Here's how the part is built. I have some questions about the finished solid (model axes, mm). Face numbers are marked on the shaded views. A direction names the side the tool comes from. Coordinates: 2 decimals unless noted, no trailing zeros. Write each loop counter-clockwise with the first axis right and the second up, starting at its lowest first coordinate (ties: lowest second). Pieces come first, ordered by that corner, then holes.
(1) Thinking about a two-plate mould opening in X: for the marked faces 1, 2, 3 and 4, which applies, released by +X, released by -X, zero draft, split by the parting line, or undercut?
(2) Imagine slicing it at C-C, the plane y = 8. List the corners of the cut face in (x, z) for me, plus the area to 3 significant figures.
(3) For pin 1 Ø0.8 at (x, z) = (-15.5, 1.5) entering from -Y; pin 2 Ø0.8 at (y, z) = (-23, 1.5) entering from -X, each with a flat end and sliding along its axis, tell me the tip position at first contact or that it passes through.
(4) Imagine slicing it at D-D, the plane x = -14. List the corners of the cut face in (y, z) for me.
(5) Please list where these lines run through material, in increasing order: probe 1 along Y at (x, z) = (0, 1.35); probe 2 along X at (y, z) = (-25, 1.8); probe 3 along Y at (x, z) = (4, 1.9).
(6) Which directions (+Z, -Z, +X, -X, +Y, -Y) give clear straight access to the entire face, cutting with the end or side of a thin tool? Please do the marked faces 5, 6 and 7.
(7) Imagine slicing it at A-A, the plane z = 1.1. List the corners of the cut face in (x, y) for me.
(8) Imagine slicing it at B-B, the plane x = 0. List the corners of the cut face in (y, z) for me.
Autodesk Inventor part; units mm, degrees
ref_plane "YZ Plane" through (0, 0, 0) normal (1, 0, 0) x (0, 1, 0)
ref_plane "XZ Plane" through (0, 0, 0) normal (0, 1, 0) x (-1, 0, 0)
ref_plane "XY Plane" through (0, 0, 0) normal (0, 0, 1) x (1, 0, 0)
sketch "Sketch1" plane through (0, 0, 0) normal (0, 0, 1) x (1, 0, 0)
  line L0 (0, 0) -> (0, 25.4)
  line L1 (0, 0) -> (0, -25.4)
  line L2 (-19.0266, -7.6091) -> (19.0734, -7.6091)
  circle A0 centre (0, 0) radius 2.54
  circle A1 centre (0, 25.4) radius 2.54
  circle A2 centre (-19.0266, -7.6091) radius 2.54
  circle A3 centre (19.0734, -7.6091) radius 2.54
  circle A4 centre (0, -25.4) radius 2.54
  circle A5 centre (0.0234, -7.6091) radius 5.08
  arc A6 (-1.9812, -2.9413) -> (-1.7729, -1.8189) centre (-2.2521, -2.3105) ccw
  arc A7 (1.7485, -1.8423) -> (1.9483, -2.9079) centre (2.1929, -2.3105) ccw
  line L3 (-2.54, 25.4) -> (-2.54, 10.1709)
  line L4 (2.54, 25.4) -> (2.54, 10.1709)
  line L5 (-2.54, -25.4) -> (-2.54, -19.0391)
  line L6 (2.54, -25.4) -> (2.54, -19.0391)
  line L7 (19.0734, -10.1491) -> (11.43, -10.1491)
  line L8 (19.0734, -5.0691) -> (17.78, -5.0691)
  line L9 (-19.0266, -5.0691) -> (-17.78, -5.0691)
  line L10 (-19.0266, -10.1491) -> (-11.43, -10.1491)
  arc A8 (-17.78, -5.0691) -> (-2.54, 10.1709) centre (-17.78, 10.1709) ccw
  arc A9 (2.54, 10.1709) -> (17.78, -5.0691) centre (17.78, 10.1709) ccw
  arc A10 (-2.54, -19.0391) -> (-11.43, -10.1491) centre (-11.43, -19.0391) ccw
  arc A11 (11.43, -10.1491) -> (2.54, -19.0391) centre (11.43, -19.0391) ccw
  circle A12 centre (-19.0266, -7.6091) radius 1.27
  circle A13 centre (0, 25.4) radius 1.27
  circle A14 centre (19.0734, -7.6091) radius 1.27
  dimension "d0" = 25.4
  dimension "d1" = 25.4
  dimension "d2" = 38.1
  dimension "d3" = 38.1
  dimension "d5" = 5.08
  dimension "d6" = 5.08
  dimension "d7" = 5.08
  dimension "d8" = 5.08
  dimension "d9" = 7.6091
  dimension "d10" = 5.08
  dimension "d12" = 4.445
  dimension "d13" = 35.56
  dimension "d14" = 22.86
  dimension "d15" = 10.16
  dimension "d16" = 2.54
  dimension "d17" = 2.54
  dimension "d18" = 2.54
extrude "Extrusion1" add sketch "Sketch1" along normal blind 2.54 contours A0 A6 A5 L2 A2 L9 A8 L3 A1 L0 | L0 A1 L4 A9 L8 A3 L2 A5 A7 A0 | A1 | A5 L1 A4 L5 A10 L10 A2 L2 | A5 L2 A3 L7 A11 L6 A4 L1 | A2 | A4 | A3
properties part number "Fish Rib"
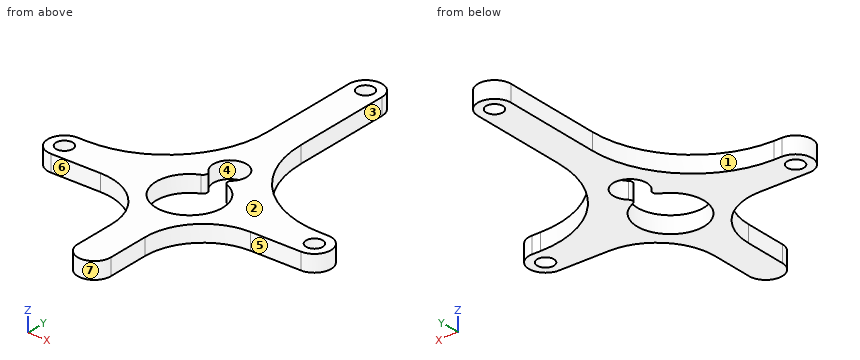
Recorded:
1. face 1: released by -X
1. face 2: zero draft
1. face 3: released by +X
1. face 4: undercut
2. outline: (-2.7, 0) - (2.7, 0) - (2.7, 2.54) - (-2.7, 2.54) - close
2. area: 13.7 mm2
3. pin 1: stops at y = -10.15
3. pin 2: stops at x = -2.54
4. outline: (-10.15, 0) - (-4.59, 0) - (-4.59, 2.54) - (-10.15, 2.54) - close
5. probe 1: y = -27.94 to -12.69, 2.54 to 24.13, 26.67 to 27.94
5. probe 2: x = -2.54 to 2.54
5. probe 3: y = -14.16 to -10.77, -4.45 to 3.66
6. face 5: +Z, -Z, +X, -Y
6. face 6: +Z, -Z, -X, -Y
6. face 7: +Z, -Z, -Y
7. outline: (-19.03, -10.15) - (-11.43, -10.15) arc R8.89 cw to (-2.54, -19.04) - (-2.54, -25.4) arc R2.54 ccw to (2.54, -25.4) - (2.54, -19.04) arc R8.89 cw to (11.43, -10.15) - (19.07, -10.15) arc R2.54 ccw to (19.07, -5.07) - (17.78, -5.07) arc R15.24 cw to (2.54, 10.17) - (2.54, 25.4) arc R2.54 ccw to (-2.54, 25.4) - (-2.54, 10.17) arc R15.24 cw to (-17.78, -5.07) - (-19.03, -5.07) arc R2.54 ccw to start; hole circle Ø2.54 at (-19.03, -7.61); hole (-1.98, -2.94) arc R5.08 ccw (long way) to (1.95, -2.91) arc R0.65 cw to (1.75, -1.84) arc R2.54 ccw (long way) to (-1.77, -1.82) arc R0.69 cw to start; hole circle Ø2.54 at (0, 25.4); hole circle Ø2.54 at (19.07, -7.61)
8. outline: (-27.94, 0) - (-12.69, 0) - (-12.69, 2.54) - (-27.94, 2.54) - close; (2.54, 0) - (24.13, 0) - (24.13, 2.54) - (2.54, 2.54) - close; (26.67, 0) - (27.94, 0) - (27.94, 2.54) - (26.67, 2.54) - close
